The model under review builds one solid part; all positions refer to its coordinate system, in mm. A direction names the side the tool comes from. Round coordinates to 2 decimals unless told otherwise and drop trailing zeros. Order: outer loops, then holes, each group sorted by start corner. A loop starts at its lowest first (then second) coordinate and runs counter-clockwise, first axis right, second up. Notation, with made-up numbers: M 67.25,-37 L 95.25,-37 A30 ccw 95.25,-6 Z; hole C 24,31.5 d7. An arc over 180 degrees is marked long. Answer as a JSON object with one key per item and string values. Group by question number.
1. Add section A-A on y = 2. State the section outline as (x, z) points.
2. Clearance check with flat-ended pins moving along their axes: P1, Ø9, axis at x = -2.5, y = 29, coming from the -Z side; P2, Ø4, axis at x = 0.5, y = 28.5, coming from the +Z side; P3, Ø12, axis at y = -26.5, z = 6, coming from the +X side. State where each tip first meets the part, or that it passes through.
3. To check wall thickness, follow probe 1 along X at (y, z) = (-74, -35); probe 2 along Y at (x, z) = (-1, -24); probe 3 along Z at (x, y) = (-25.5, -37.5). State the ranges of each line that lie inside material, in increasing order. Write a range as [from, to].
4. Machinability: for faces 5 (the face through (0, 28, 1)), 6 (the face through (-25, -43, -26)), 7 (the face through (-6, -74, -33)), 8 (the face through (-19, 13, -7)), which of the approach directions +Z, -Z, +X, -X, +Y, -Y give a long, thin tool a straight path to every point of the face, cutting with its end or side? Answer none if there is none.
5. Add section D-D on y = -65.5. State the section outline as (x, z) points.
6. Mouldability with a two-part tool opening along Z and no side actions: class faces 1 (the face through (0, 23, 9)), 2 (the face through (0, 28, -15)), 3 (the face through (-3, -25, -2)), 4 (the face through (-7, -15, -38)) as released by +Z, released by -Z, zero draft, split by the parting line, or undercut.
7. Add section B-B on x = -25. State the section outline as (y, z) points, and give its area (3 significant figures).
8. Add section C-C on z = -7. State the section outline as (x, y) points, and give its area (3 significant figures).
```python
from build123d import *

# Parameters (mm, degrees)
SKETCH1_R                = 19
BOSS_EXTRUDE1_DEPTH      = 38
BOSS_EXTRUDE2_DEPTH      = 2
BOSS_EXTRUDE2_DEPTH_BACK = 12
BOSS_EXTRUDE3_START      = -10
BOSS_EXTRUDE3_DEPTH      = 10
BOSS_EXTRUDE4_DEPTH      = 19
HOLE1_D                  = 16
HOLE1_DEPTH              = 100
HOLE2_D                  = 19
HOLE2_DEPTH              = 100
BOSS_EXTRUDE5_DEPTH      = 3


with BuildPart() as part:
    # Sketch1 → Boss-Extrude1 (new, symmetric)
    with BuildSketch(Plane.XY):
        Circle(SKETCH1_R)
    extrude(amount=BOSS_EXTRUDE1_DEPTH, both=True)



with BuildPart() as body_2:
    # Sketch2 → Boss-Extrude2 (new, two sides: drawn at the far end of the back side and taken through both)
    with BuildSketch(Plane(origin=(0, 0, -38), x_dir=(-1, 0, 0), z_dir=(0, 0, -1)).offset(-BOSS_EXTRUDE2_DEPTH_BACK)):
        with BuildLine():
            Line((6, -64), (6, -85.242645786))
            ThreePointArc((6, -85.242645786), (25, -35.5), (44, -85.242645786))
            Line((44, -85.242645786), (44, -64))
            ThreePointArc((44, -64), (25, -45), (6, -64))
        make_face()
    extrude(amount=BOSS_EXTRUDE2_DEPTH + BOSS_EXTRUDE2_DEPTH_BACK)


with BuildPart() as part_1:
    add(part.part)

    add(body_2.part)  # Boss-Extrude3 merges body 2
    # Sketch3 → Boss-Extrude3 (add)
    with BuildSketch(Plane(origin=(0, 0, -38), x_dir=(-1, 0, 0), z_dir=(0, 0, -1)).offset(BOSS_EXTRUDE3_START)):
        with BuildLine():
            Line((-18.483548174, -4.399823506), (-2.725322262, -70.599735258))
            ThreePointArc((-2.725322262, -70.599735258), (14.630259976, -37.45346554), (49.857815378, -50.059447118))
            Line((49.857815378, -50.059447118), (16.571876918, 9.293701921))
            ThreePointArc((16.571876918, 9.293701921), (6.913160016, -17.69768964), (-18.483548174, -4.399823506))
        make_face()
    extrude(amount=BOSS_EXTRUDE3_DEPTH)

    # Sketch4 → Boss-Extrude4 (add, symmetric)
    with BuildSketch(Plane(origin=(0, 0, 0), x_dir=(0, 0, -1), z_dir=(1, 0, 0))):
        with BuildLine():
            Line((-9, 0), (-9, 32))
            Line((-9, 32), (-1, 32))
            Line((-1, 32), (-1, 24))
            ThreePointArc((-1, 24), (7, 16), (15, 24))
            Line((15, 24), (15, 32))
            Line((15, 32), (23, 32))
            Line((23, 32), (23, 0))
            Line((23, 0), (-9, 0))
        make_face()
    extrude(amount=BOSS_EXTRUDE4_DEPTH, both=True)

    # Hole1
    with Locations(Plane(origin=(19, 0, 0), x_dir=(0, 0, -1), z_dir=(1, 0, 0))):
        with Locations((7, 24)):
            Hole(HOLE1_D / 2, depth=HOLE1_DEPTH)

    # Hole2
    with Locations(Plane.XY.offset(38)):
        with Locations((0, 0)):
            Hole(HOLE2_D / 2, depth=HOLE2_DEPTH)

    # Sketch10 → Boss-Extrude5 (add, symmetric)
    with BuildSketch(Plane(origin=(0, 0, 0), x_dir=(0, 0, -1), z_dir=(1, 0, 0))):
        Polygon((-38, -19), (28, -34), (30, -34), (30, -17), (-38, -17), align=None)
    extrude(amount=BOSS_EXTRUDE5_DEPTH, both=True)


solid = part_1.part
```
Recorded:
{
 "1": {"outline": "M -20.66,-38 L -9.29,-38 L -9.29,38 L -18.89,38 L -18.89,9 L -19,9 L -19,-23 L -18.89,-23 L -18.89,-28 L -20.66,-28 Z; M 9.29,-38 L 18.89,-38 L 18.89,-23 L 19,-23 L 19,9 L 18.89,9 L 18.89,38 L 9.29,38 Z"},
 "2": {"P1": "stops at z = -23", "P2": "stops at z = 9", "P3": "stops at x = 3"},
 "3": {"probe 1": "x = [-51.69, -44], [-6, 1.69]", "probe 2": "y = [-33.09, -9.45], [9.45, 18.97]", "probe 3": "z = [-40, -26]"},
 "4": {"face 5": "+X, -X, +Y", "face 6": "+Z, +X, -X, -Y", "face 7": "+Z, -Z, -Y", "face 8": "+Z, -X, +Y, -Y"},
 "5": {"outline": "M -53.46,-40 L -44,-40 L -44,-26 L -53.46,-26 Z; M -6,-40 L 3.46,-40 L 3.46,-38 L 3.94,-38 L 3.94,-28 L 3.46,-28 L 3.46,-26 L -6,-26 Z"},
 "6": {"face 1": "released by +Z", "face 2": "undercut", "face 3": "zero draft", "face 4": "released by -Z"},
 "7": {"outline": "M -45,-40 L -35.5,-40 L -35.5,-38 L -5.73,-38 L -5.73,-28 L -35.5,-28 L -35.5,-26 L -45,-26 Z", "area": "431 mm²"},
 "8": {"outline": "M -19,0 A19 ccw -3,-18.76 L -3,-29.23 L 3,-29.23 L 3,-18.76 A19 ccw 19,0 L 19,16 L -19,16 Z; hole C 0,0 d19", "area": "953 mm²"}
}
